```python
from build123d import *

# Parameters (mm, degrees)
F0_R     = 101.6
F0_R_2   = 19.05
F1_DEPTH = 25.4
F2_R     = 19.05
F3_DEPTH = 5.08
F5_DEPTH = 63.5


with BuildPart() as f1:
    # F0 (on Top) → F1 (new body)
    with BuildSketch(Plane.XY):
        Circle(F0_R)
        with BuildLine():
            ThreePointArc((19.05, -50.8), (-13.4703841816, -64.2703841816), (0, -31.75))
            ThreePointArc((0, -31.75), (13.4703841816, -37.3296158184), (19.05, -50.8))
        make_face(mode=Mode.SUBTRACT)
        with Locations((-50.8, 0)):
            Circle(F0_R_2, mode=Mode.SUBTRACT)
        with BuildLine():
            ThreePointArc((69.85, 0), (50.8, -19.05), (31.75, 0))
            ThreePointArc((31.75, 0), (50.8, 19.05), (69.85, 0))
        make_face(mode=Mode.SUBTRACT)
        with BuildLine():
            ThreePointArc((19.05, 50.8), (13.4703841816, 37.3296158184), (0, 31.75))
            ThreePointArc((0, 31.75), (-13.4703841816, 64.2703841816), (19.05, 50.8))
        make_face(mode=Mode.SUBTRACT)
    extrude(amount=F1_DEPTH)

    # F2 (on Top) → F3 (join)
    with BuildSketch(Plane.XY):
        with Locations((-50.8, 0)):
            Circle(F2_R)
        with Locations((0, -50.8)):
            Circle(F2_R)
        with Locations((0, 50.8)):
            Circle(F2_R)
        with Locations((50.8, 0)):
            Circle(F2_R)
    extrude(amount=F3_DEPTH)

    # F4 (on face) → F5 (join)
    with BuildSketch(Plane.XY.offset(25.4)):
        Polygon((-45.4118463274, 32.3289220358), (-31.9414621458, 18.8585378542), (32.3289220358, -45.4118463274), (35.9210244843, -41.8197438789), (-41.8197438789, 35.9210244843), align=None)
        Polygon((46.7480724009, -30.9926959623), (-18.5676223436, 34.3229987821), (-30.9926959623, 46.7480724009), (-34.5847984107, 43.1559699525), (43.1559699525, -34.5847984107), align=None)
    extrude(amount=F5_DEPTH)


solid = f1.part
```
Could you check a few things on this model? Use its own coordinates, in mm. A direction names the side the tool comes from. Round coordinates to 2 decimals unless told otherwise and drop trailing zeros. Write each loop counter-clockwise with the first axis right and the second up, starting at its lowest first coordinate (ties: lowest second). Pieces come first, ordered by that corner, then holes. Notation, with made-up numbers: M -36.75,20.25 L 4.25,20.25 A30 cw 4.25,52.25 Z; hole C -10,73.5 d8. An arc over 180 degrees is marked long. Answer in a Markdown table with one row per item. Add a question column.
Q1. Imagine slicing it at B-B (z = 10). Please give me the cut outline in (x, y), then the cut area to 3 significant figures.
Q2. On a 3-axis mill with a long thin cutter (end or side, diameter ignored), from which of +Z, -Z, +X, -X, +Y, -Y can I reach the whole of each face in a straight line? I mean faces 4 (the cylindrical face through (-22.025, -99.184, 12.522)), 5 (the flat face through (51, 0, 5.08)). Say none if no direction works.
Q3. If I drill on line 1 (Z direction, x = 77, y = 28); line 2 (Z direction, x = 15, y = 50.5); line 3 (X direction, y = 6.5, z = 24), over which ranges is the centre line in solid material (lowest first)? Write a range as from..to.
Q4. Imagine slicing it at C-C (y = -55.5). Please give me the cut outline in (x, z), then the cut area to 3 significant figures.
Q5. Will these pins go through, and if not, where does the flat tip stop? pin 1 Ø23 at (x, y) = (0, -50.8) entering from +Z; pin 2 Ø2 at (y, z) = (-19.5, 27.5) entering from +X; pin 3 Ø5 at (x, y) = (61.5, 24) entering from +Z.
Q6. Imagine slicing it at A-A (z = 28). Please give me the cut outline in (x, y), then the cut area to 3 significant figures.
Q7. If we mould it in two halves opening along Y, with no side actions, what happens to faces 1 (the flat face through (-7.086, -5.997, 56.706)), 2 (the flat face through (0, 51, 5.08)), 3 (the flat face through (-5, -5, 88.9))? For each: +Y half, -Y half, draft (parallel to the pull), parting line (faces both ways), or undercut.
Q8. Imagine slicing it at D-D (x = 50.8). Please give me the cut outline in (y, z), then the cut area to 3 significant figures.
Values:
| question | item | result |
|---|---|---|
| 1 | outline | C 0,0 d203.2; hole C -50.8,0 d38.1; hole C 0,-50.8 d38.1; hole C 0,50.8 d38.1; hole C 50.8,0 d38.1 |
| 1 | area | 27,900 mm^2 |
| 2 | face 4 | +Z, -Z |
| 2 | face 5 | +Z |
| 3 | line 1 | 0..25.4 |
| 3 | line 2 | 0..5.08 |
| 3 | line 3 | -101.39..-68.71, -32.89..32.89, 68.71..101.39 |
| 4 | outline | M -85.1,0 L 85.1,0 L 85.1,25.4 L 18.46,25.4 L 18.46,5.08 L -18.46,5.08 L -18.46,25.4 L -85.1,25.4 Z |
| 4 | area | 3,570 mm^2 |
| 5 | pin 1 | z = 5.08 |
| 5 | pin 2 | x = 36.26 |
| 5 | pin 3 | z = 25.4 |
| 6 | outline | M -45.41,32.33 L 32.33,-45.41 L 35.92,-41.82 L -41.82,35.92 Z; M -34.58,43.16 L 43.16,-34.58 L 46.75,-30.99 L -30.99,46.75 Z |
| 6 | area | 1,120 mm^2 |
| 7 | face 1 | -Y half |
| 7 | face 2 | undercut |
| 7 | face 3 | draft |
| 8 | outline | M -87.99,0 L 87.99,0 L 87.99,25.4 L 19.05,25.4 L 19.05,5.08 L -19.05,5.08 L -19.05,25.4 L -87.99,25.4 Z |
| 8 | area | 3,700 mm^2 |
